Geometry: see drawing. Coordinates: mm, zero at the bounding-box minimum. A direction names the side the tool comes from. Coordinates: 2 decimals unless noted, no trailing zeros. Order: outer loops, then holes, each group sorted by start corner. A loop starts at its lowest first (then second) coordinate and runs counter-clockwise, first axis right, second up.
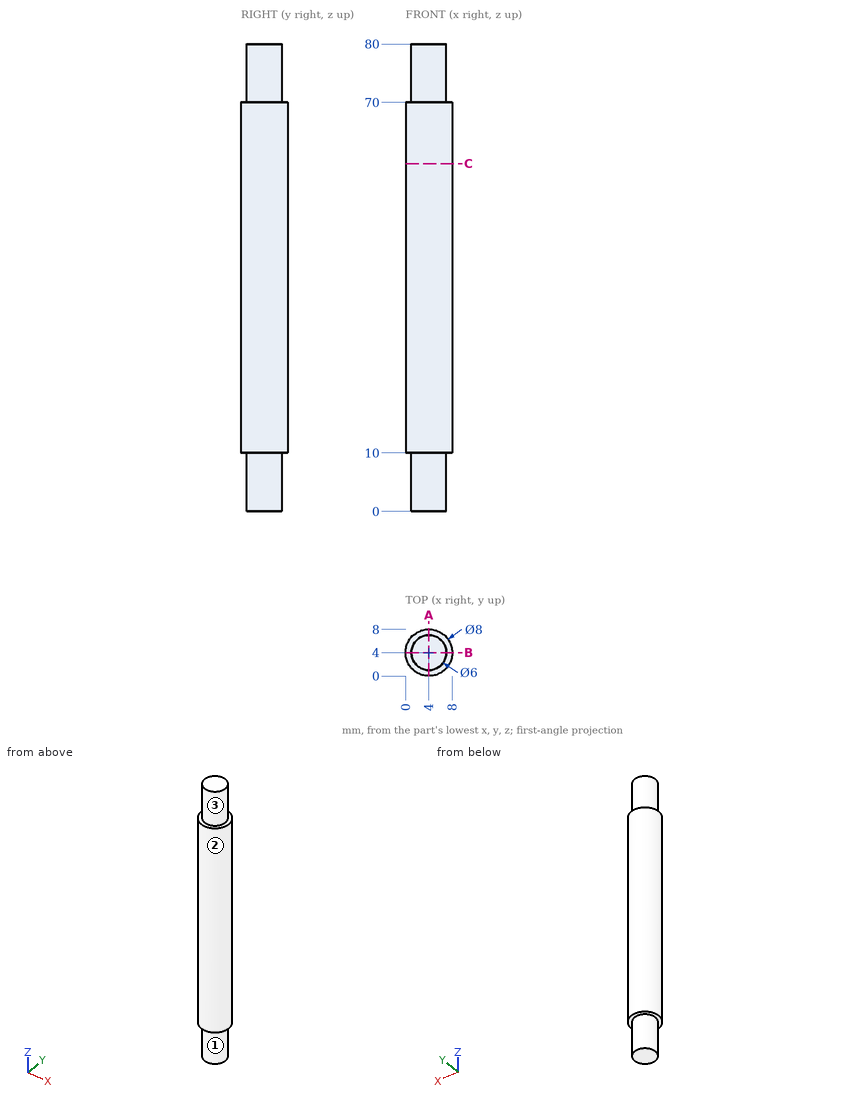
Q1. Material intervals for line 1 along Z through (x, y) = (7, 6.5); line 2 along Y through (x, z) = (4.25, 7.5); line 3 along Y through (x, z) = (5.75, 31), sorted ascending.
Solutions:
line 1: z = 10 to 70
line 2: y = 1.01 to 6.99
line 3: y = 0.4 to 7.6
Q2. Section query A-A on x = 4. Output: boundary loops of the cut face in (y, z), plus the area to 3 significant figures.
Solutions:
outline: (0, 10) - (1, 10) - (1, 0) - (7, 0) - (7, 10) - (8, 10) - (8, 70) - (7, 70) - (7, 80) - (1, 80) - (1, 70) - (0, 70) - close
area: 600 mm2
Q3. Section query C-C on z = 59.5. Output: boundary loops of the cut face in (x, y), plus the area to 3 significant figures.
Solutions:
outline: circle Ø8 at (4, 4)
area: 50.3 mm2
Q4. Pin query (flat end, axial travel): P1, Ø1, axis at y = 5.5, z = 66, coming from the -X side; P2, Ø3, axis at y = 1, z = 56, coming from the +X side. Return the tip coordinate at first contact, or that it passes through.
Solutions:
P1: stops at x = 0.13
P2: stops at x = 7.71
Q5. Set-up query: the marked faces 1, 2 and 3. Return all of +Z, -Z, +X, -X, +Y, -Y with unobstructed straight access to the full face (end or side cutting, diameter ignored); none if empty.
Solutions:
face 1: -Z
face 2: +Z, -Z
face 3: +Z
